```python
from build123d import *

# Parameters (mm, degrees)
SKETCH_2_W          = 30
SKETCH_2_H          = 14
SKETCH_2_R          = 5.1
EXTRUDE_1_DEPTH     = 40
SKETCH_3_R          = 2
CUT_EXTRUDE_1_DEPTH = 52.923019943


with BuildPart() as part:
    # 草圖2 → 填料-伸長1 (new body)
    with BuildSketch(Plane(origin=(0, 0, 0), x_dir=(0, 0, -1), z_dir=(1, 0, 0))):
        with Locations((15, 7)):
            Rectangle(SKETCH_2_W, SKETCH_2_H)
        with Locations((15, 7)):
            Circle(SKETCH_2_R, mode=Mode.SUBTRACT)
    extrude(amount=EXTRUDE_1_DEPTH)

    # 草圖3 → 除料-伸長1 (cut, through all)
    with BuildSketch(Plane(origin=(0, 14, 0), x_dir=(1, 0, 0), z_dir=(0, 1, 0))):
        with Locations(Location((20, 15, 0), (0, 0, 270))):
            Circle(SKETCH_3_R)
    extrude(amount=-CUT_EXTRUDE_1_DEPTH, mode=Mode.SUBTRACT)


solid = part.part
```
For this review, take the finished solid that the model builds, in its own axes (mm). Round coordinates to 2 decimals unless told otherwise and drop trailing zeros. Loops run counter-clockwise (first coordinate to the right, second up) from the corner with the lowest first, then second, coordinate; pieces in that order, holes last.
Q1. Add section D-D on x = 35. Write out the cut boundary in (y, z).
Result sheet:
outline: (0, -30) - (14, -30) - (14, 0) - (0, 0) - close; hole circle Ø10.2 at (7, -15)
Q2. Add section C-C on z = -15. Write out the cut boundary in (x, y).
Result sheet:
outline: (0, 0) - (18, 0) - (18, 1.9) - (0, 1.9) - close; (0, 12.1) - (18, 12.1) - (18, 14) - (0, 14) - close; (22, 0) - (40, 0) - (40, 1.9) - (22, 1.9) - close; (22, 12.1) - (40, 12.1) - (40, 14) - (22, 14) - close
Q3. To check wall thickness, follow line 1 along Y through (x, z) = (25, -15); line 2 along Z through (x, y) = (20, 12.5); line 3 along X through (y, z) = (12.8, -15). State the ranges of each line that lie inside material, in increasing order.
Result sheet:
line 1: y = 0 to 1.9, 12.1 to 14
line 2: z = -30 to -17, -13 to 0
line 3: x = 0 to 18, 22 to 40
Q4. Add section A-A on x = 20. Write out the cut boundary in (y, z).
Result sheet:
outline: (0, -30) - (14, -30) - (14, -17) - (11.69, -17) arc R5.1 cw to (2.31, -17) - (0, -17) - close; (0, -13) - (2.31, -13) arc R5.1 cw to (11.69, -13) - (14, -13) - (14, 0) - (0, 0) - close
Q5. Add section B-B on y = 7. Write out the cut boundary in (x, z).
Result sheet:
outline: (0, -30) - (40, -30) - (40, -20.1) - (0, -20.1) - close; (0, -9.9) - (40, -9.9) - (40, 0) - (0, 0) - close
Q6. Mouldability with a two-part tool opening along Y and no side actions: class faces 1 (the face through (19.72, 8.532, -19.864)), 2 (the face through (20, 7, 0)), 3 (the face through (20, 0, -11)) as +Y half, -Y half, draft (parallel to the pull), parting line (faces both ways), or undercut.
Result sheet:
face 1: undercut
face 2: draft
face 3: -Y half
